from build123d import *

# Parameters (mm, degrees)
CROQUIS1_W              = 240
CROQUIS1_H              = 70
SALIENTE_EXTRUIR1_DEPTH = 5
CROQUIS2_R              = 2.25
CORTAR_EXTRUIR1_DEPTH   = 126.39936204


with BuildPart() as part:
    # Croquis1 → Saliente-Extruir1 (new, symmetric)
    with BuildSketch(Plane(origin=(0, 0, 0), x_dir=(1, 0, 0), z_dir=(0, 1, 0))):
        Rectangle(CROQUIS1_W, CROQUIS1_H)
    extrude(amount=SALIENTE_EXTRUIR1_DEPTH, both=True)

    # Croquis2 → Cortar-Extruir1 (cut, through all)
    with BuildSketch(Plane(origin=(0, 5, 0), x_dir=(1, 0, 0), z_dir=(0, 1, 0))):
        with Locations(Location((-115, 20, 0), (0, 0, 270))):
            Circle(CROQUIS2_R)
        with Locations(Location((-115, -20, 0), (0, 0, 270))):
            Circle(CROQUIS2_R)
        with Locations(Location((115, -20, 0), (0, 0, 90))):
            Circle(CROQUIS2_R)
        with Locations(Location((115, 20, 0), (0, 0, 90))):
            Circle(CROQUIS2_R)
    extrude(amount=-CORTAR_EXTRUIR1_DEPTH, mode=Mode.SUBTRACT)


solid = part.part
Could you check a few things on this model? Use its own coordinates, in mm. Give positions to 0.01 mm unless a question says otherwise; leave off trailing zeros. Order: outer loops, then holes, each group sorted by start corner. A loop starts at its lowest first (then second) coordinate and runs counter-clockwise, first axis right, second up. Notation, with made-up numbers: (89.25, 69) - (100.25, 69) arc R25 ccw to (100.25, 98) - close; hole circle Ø9 at (-35, 41.5). An arc over 180 degrees is marked (long way). Return JSON: item names as keys, results as strings. Group by question number.
Q1. Please list where these lines run through material, in increasing order: line 1 along Z through (x, y) = (115, 0.5); line 2 along X through (y, z) = (-0.75, -20). Write a range as [from, to].
Q2. Suppose I cut it at A-A, the plane x = 115. Please give me the cut outline in (y, z).
Q3. Suppose I cut it at B-B, the plane z = 20. Please give me the cut outline in (x, y), and give its area (3 significant figures).
Q4. Will these pins go through, and if not, where does the flat tip stop? pin 1 Ø5 at (x, z) = (115, 20) entering from -Y; pin 2 Ø2.5 at (x, z) = (-115, 20) entering from -Y.
Q5. Thinking about a two-plate mould opening in Z: for faces 1 (the face through (-2, 0, 35)), 2 (the face through (-2, -5, 0)), 3 (the face through (-117.196, 0.07, -20.488)), which applies, pulls with the +Z half, pulls with the -Z half, needs draft (parallel to the pull), parting line crosses it, or undercut?
Resolved:
{
 "1": {"line 1": "z = [-35, -22.25], [-17.75, 17.75], [22.25, 35]", "line 2": "x = [-120, -117.25], [-112.75, 112.75], [117.25, 120]"},
 "2": {"outline": "(-5, -35) - (5, -35) - (5, -22.25) - (-5, -22.25) - close; (-5, -17.75) - (5, -17.75) - (5, 17.75) - (-5, 17.75) - close; (-5, 22.25) - (5, 22.25) - (5, 35) - (-5, 35) - close"},
 "3": {"outline": "(-120, -5) - (-117.25, -5) - (-117.25, 5) - (-120, 5) - close; (-112.75, -5) - (112.75, -5) - (112.75, 5) - (-112.75, 5) - close; (117.25, -5) - (120, -5) - (120, 5) - (117.25, 5) - close", "area": "2,310 mm2"},
 "4": {"pin 1": "stops at y = -5", "pin 2": "passes through"},
 "5": {"face 1": "pulls with the +Z half", "face 2": "needs draft", "face 3": "undercut"}
}
